```python
from build123d import *

# Parameters (mm, degrees)
F0_W     = 136.525
F0_H     = 66.675
F1_DEPTH = 47.625
F3_DEPTH = 25.4
F4_DEPTH = 68.2625


with BuildPart() as f1:
    # F0 (on Front) → F1 (new body)
    with BuildSketch(Plane.XZ):
        with Locations((68.2625, 33.3375)):
            Rectangle(F0_W, F0_H)
    extrude(amount=F1_DEPTH)

    # F2 (on face) → F3 (cut)
    with BuildSketch(Plane.XZ.offset(47.625)):
        Polygon((117.475, 66.675), (19.05, 66.675), (56.3245, 0), (80.2005, 0), align=None)
    extrude(amount=-F3_DEPTH, mode=Mode.SUBTRACT)

    # F4 (cut): a face of the model
    f4_faces = [f1.faces().sort_by_distance(p)[0] for p in [
        (0, -23.8125, 33.3375),
    ]]
    extrude(f4_faces, amount=-F4_DEPTH, mode=Mode.SUBTRACT)


solid = f1.part
```
Can you work these out from the model? Positions are in its coordinate system, mm. A direction names the side the tool comes from. Coordinates: 2 decimals unless noted, no trailing zeros. Loops run counter-clockwise (first coordinate to the right, second up) from the corner with the lowest first, then second, coordinate; pieces in that order, holes last. Notation, with made-up numbers: (23, 71.5) - (38, 71.5) arc R20 cw to (38, 94.5) - close; hole circle Ø10 at (-37.5, -38.75). An arc over 180 degrees is marked (long way). Answer as CSV lines item,"result". Start each with the question number.
1) Suppose I cut it at C-C (y = -41). Please give me the cut outline in (x, z) (1 decimal), plus the area to 3 significant figures.
2) Suppose I cut it at A-A (z = 44.5). Please give me the cut outline in (x, y) (1 decimal).
3) Suppose I cut it at D-D (x = 77). Please give me the cut outline in (y, z) (3 decimals), plus the area to 3 significant figures.
4) For pin 1 (10 mm diameter, centred on x = 83.5, y = -37.5, fed in from +Z); pin 2 (15 mm diameter, centred on x = 93, z = 42, fed in from -Y) (3 decimals); pin 3 (1.5 mm diameter, centred on y = -35.5, z = 14.5, fed in from -X), each with a flat end and sliding along its axis, tell me the tip position at first contact or that it passes through.
5) Which directions (+Z, -Z, +X, -X, +Y, -Y) give clear straight access to the entire face, cutting with the end or side of a thin tool? Please do faces 1 (the flat face through (98.577, -35.103, 32.871)), 2 (the flat face through (102, 0, 34)).
6) Suppose I cut it at B-B (x = 92.5). Please give me the cut outline in (y, z) (3 decimals), plus the area to 3 significant figures.
7) I need wall thicknesses on line 1 (Y direction, x = 87, z = 44) (3 decimals); line 2 (X direction, y = -44, z = 7) (3 decimals); line 3 (Z direction, x = 91, y = -26.5). Which ranges of each line are inside material? Lowest first, please. Write a range as from..to.
Check result:
1,outline,"(80.2, 0) - (136.5, 0) - (136.5, 66.7) - (117.5, 66.7) - close"
1,area,"2,510 mm²"
2,outline,"(68.3, -22.2) - (105.1, -22.2) - (105.1, -47.6) - (136.5, -47.6) - (136.5, 0) - (68.3, 0) - close"
3,outline,"(-22.225, 0) - (0, 0) - (0, 66.675) - (-22.225, 66.675) - close"
3,area,"1,480 mm²"
4,pin 1,"stops at z = 14.85"
4,pin 2,"stops at y = -22.225"
4,pin 3,"stops at x = 87.89"
5,face 1,"+Z, -X, -Y"
5,face 2,"+Z, -Z, +X, -X, +Y"
6,outline,"(-47.625, 0) - (0, 0) - (0, 66.675) - (-22.225, 66.675) - (-22.225, 22.001) - (-47.625, 22.001) - close"
6,area,"2,040 mm²"
7,line 1,"y = -22.225..0"
7,line 2,"x = 84.114..136.525"
7,line 3,"z = 0..19.32"
